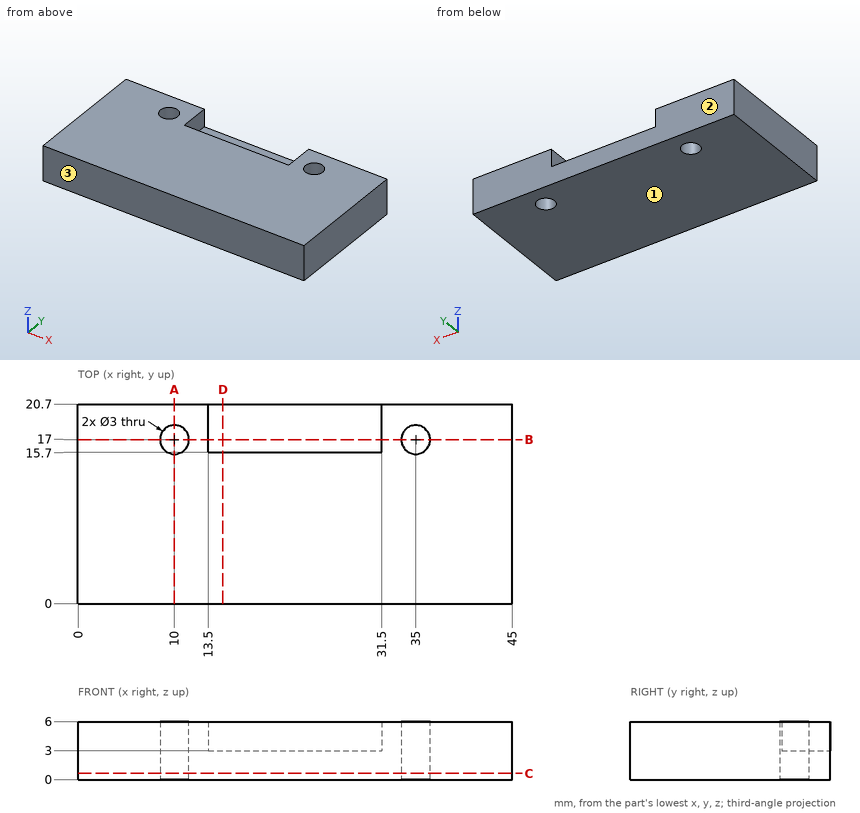
Geometry check sheet. Reference: drawing and pictorial views, mm from the part's lowest x, y, z. Give positions to 0.01 mm unless a question says otherwise; leave off trailing zeros. Loops run counter-clockwise (first coordinate to the right, second up) from the corner with the lowest first, then second, coordinate; pieces in that order, holes last. Notation, with made-up numbers: (83, 5.25) -> (105, 5.25) arc R15 ccw to (105, 21.25) -> close; hole circle Ø1 at (30.25, 52). An arc over 180 degrees is marked (long way). Answer in a Markdown table with one row per item. Add a question column.
1) Cross-section at A-A on x = 10. Record the boundary of the cut face in (y, z), and give its area (3 significant figures).
2) Cross-section at D-D on x = 15. Record the boundary of the cut face in (y, z).
3) Gauge pin test, flat ends, axial feed: P1, Ø2.5, axis at x = 35, y = 17, coming from the +Z side; P2, Ø1.5, axis at x = 22, y = 19, coming from the +Z side. Record the tip position at first contact, or that the pin passes through.
4) Cross-section at B-B on y = 17. Record the boundary of the cut face in (x, z), and give its area (3 significant figures).
5) Draft check along Y on the marked faces 1, 2 and 3. Enter one of: pulls with the +Y half, pulls with the -Y half, needs draft (parallel to the pull), parting line crosses it, or undercut.
6) Material ranges on probe 1 along Y at (x, z) = (35, 3.55); probe 2 along Z at (x, y) = (20.5, 17.5); probe 3 along X at (y, z) = (17.5, 0.4), recorded low to high. Write a range as from..to.
7) Cross-section at C-C on z = 0.65. Record the boundary of the cut face in (x, y), and give its area (3 significant figures).
Outcome:
| question | item | result |
|---|---|---|
| 1 | outline | (0, 0) -> (15.5, 0) -> (15.5, 6) -> (0, 6) -> close; (18.5, 0) -> (20.7, 0) -> (20.7, 6) -> (18.5, 6) -> close |
| 1 | area | 106 mm^2 |
| 2 | outline | (0, 0) -> (20.7, 0) -> (20.7, 3) -> (15.7, 3) -> (15.7, 6) -> (0, 6) -> close |
| 3 | P1 | passes through |
| 3 | P2 | stops at z = 3 |
| 4 | outline | (0, 0) -> (8.5, 0) -> (8.5, 6) -> (0, 6) -> close; (11.5, 0) -> (33.5, 0) -> (33.5, 6) -> (31.5, 6) -> (31.5, 3) -> (13.5, 3) -> (13.5, 6) -> (11.5, 6) -> close; (36.5, 0) -> (45, 0) -> (45, 6) -> (36.5, 6) -> close |
| 4 | area | 180 mm^2 |
| 5 | face 1 | needs draft |
| 5 | face 2 | pulls with the +Y half |
| 5 | face 3 | pulls with the -Y half |
| 6 | probe 1 | y = 0..15.5, 18.5..20.7 |
| 6 | probe 2 | z = 0..3 |
| 6 | probe 3 | x = 0..8.59, 11.41..33.59, 36.41..45 |
| 7 | outline | (0, 0) -> (45, 0) -> (45, 20.7) -> (0, 20.7) -> close; hole circle Ø3 at (10, 17); hole circle Ø3 at (35, 17) |
| 7 | area | 917 mm^2 |
